Verification items for this drawing (mm, ordinates from the low corner). A direction names the side the tool comes from. Give positions to 0.01 mm unless a question says otherwise; leave off trailing zeros. Write each loop counter-clockwise with the first axis right and the second up, starting at its lowest first coordinate (ties: lowest second). Pieces come first, ordered by that corner, then holes. Notation, with made-up numbers: (26.5, -16) -> (72.5, -16) arc R14 ccw to (72.5, 8) -> close; hole circle Ø6 at (25, 67.25). An arc over 180 degrees is marked (long way). Use one line per item in the form item = value. Start each with the question number.
(1) Section check B-B, the plane y = 44.5. Record the cut outline in (x, z), plus the area to 3 significant figures.
(2) Depth check by flat-ended pin: pin 1 Ø1 at (y, z) = (16, 33) entering from -X; pin 2 Ø8 at (y, z) = (40, 31) entering from +X (3 decimals); pin 3 Ø1 at (x, y) = (28, 29.5) entering from -Z. Enter the tip coordinate at first touch or a pass-through.
(3) Section check A-A, the plane x = 20. Record the cut outline in (y, z).
(4) Section check D-D, the plane x = 11. Record the cut outline in (y, z).
(5) Scan lines: L1, parallel to Z at x = 20, y = 43; L2, parallel to X at y = 47, z = 25.5; L3, parallel to Z at x = 34, y = 44. Record each from-to range of solid material in increasing order.
(6) Section check C-C, the plane z = 36. Record the cut outline in (x, y).
(7) Set-up check for the marked faces 1, 2 and 3: record each of +Z, -Z, +X, -X, +Y, -Y from which the full face is reachable in a straight line by a thin tool's end or side.
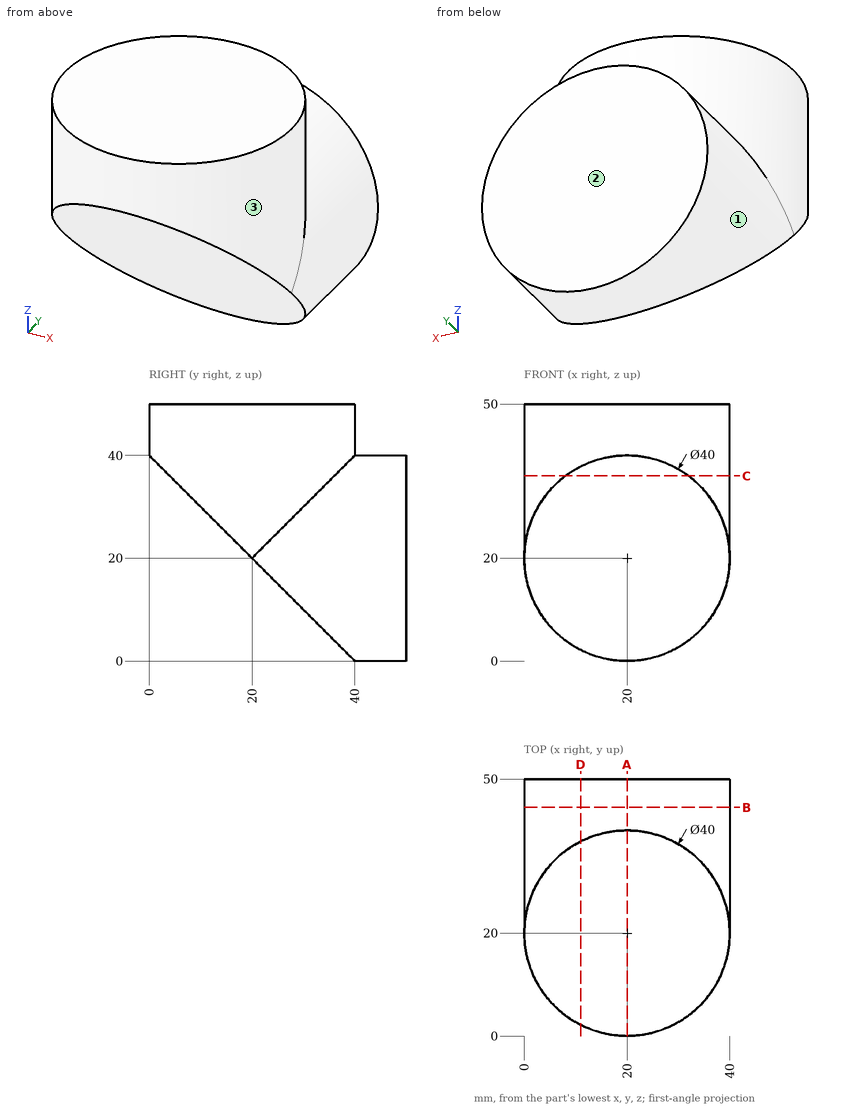
Completed:
q1.outline = circle Ø40 at (20, 20)
q1.area = 1,260 mm²
q2.pin_1 = 0.31
q2.pin_2 = 38.735
q2.pin_3 = 10
q3.outline = (0, 40) -> (40, 0) -> (50, 0) -> (50, 40) -> (40, 40) -> (40, 50) -> (0, 50) -> close
q4.outline = (2.14, 37.86) -> (37.86, 2.14) -> (50, 2.14) -> (50, 37.86) -> (37.86, 37.86) -> (37.86, 50) -> (2.14, 50) -> close
q5.L1 = 0 to 40
q5.L2 = 0.77 to 39.23
q5.L3 = 5.72 to 34.28
q6.outline = (8, 4) -> (32, 4) arc R20 ccw to (32, 36) -> (32, 50) -> (8, 50) -> (8, 36) arc R20 ccw to start
q7.face_1 = +Y
q7.face_2 = +Z, -Z, +X, -X, +Y
q7.face_3 = +Z
